Design review of the part built by this model. Coordinates are the model's own, in mm. Face numbers are marked on the shaded views. A direction names the side the tool comes from. Give positions to 0.01 mm unless a question says otherwise; leave off trailing zeros. Loops run counter-clockwise (first coordinate to the right, second up) from the corner with the lowest first, then second, coordinate; pieces in that order, holes last. Notation, with made-up numbers: M 18.5,-8 L 62.5,-8 A15 cw 62.5,17 Z; hole C 43,5 d2. An arc over 180 degrees is marked long. Use CSV: the item, a comma, the result in double quotes.
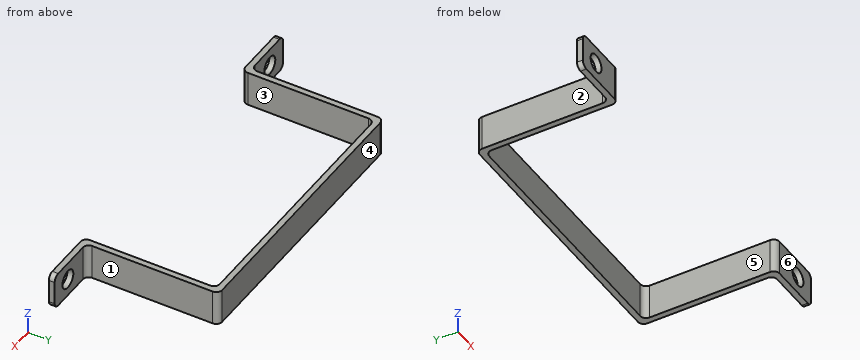
from build123d import *

# Parameters (mm, degrees)
EXTRUDE_1_DEPTH     = 12
FILLET_1_R          = 2
SKETCH_2_R          = 3.1
CUT_EXTRUDE_1_DEPTH = 12


with BuildPart() as part:
    # ｽｹｯﾁ1 → ﾎﾞｽ - 押し出し1 (new body)
    with BuildSketch(Plane.XY):
        Polygon((47, 0), (-47, 0), (-47, -45), (-65, -45), (-65, -47), (-45, -47), (-45, -2), (45, -2), (45, -47), (65, -47), (65, -45), (47, -45), align=None)
    extrude(amount=EXTRUDE_1_DEPTH)

    # ﾌｨﾚｯﾄ1
    fillet_1_edges = [part.edges().sort_by_distance(p)[0] for p in [
        (65, -46, 0),
        (-65, -46, 0),
        (-65, -46, 12),
        (45, -47, 6),
        (45, -2, 6),
        (-45, -2, 6),
        (-45, -47, 6),
        (-47, -45, 6),
        (-47, 0, 6),
        (47, 0, 6),
        (47, -45, 6),
        (65, -46, 12),
    ]]
    fillet(fillet_1_edges, radius=FILLET_1_R)

    # ｽｹｯﾁ2 → ｶｯﾄ - 押し出し1 (cut)
    with BuildSketch(Plane(origin=(0, -45, 0), x_dir=(1, 0, 0), z_dir=(0, 1, 0))):
        with Locations(Location((-57.5, -6, 0), (0, 0, 180))):
            Circle(SKETCH_2_R)
        with Locations(Location((57.5, -6, 0), (0, 0, 180))):
            Circle(SKETCH_2_R)
    extrude(amount=-CUT_EXTRUDE_1_DEPTH, mode=Mode.SUBTRACT)


solid = part.part
(1) The part is to be moulded in two halves that separate along X. For the marked faces 1, 2, 3 and 4, say which applies: released by +X, released by -X, zero draft, split by the parting line, or undercut.
A:
face 1,"released by +X"
face 2,"released by -X"
face 3,"undercut"
face 4,"zero draft"
(2) Machinability: for the marked faces 5 and 6, which of the approach directions +Z, -Z, +X, -X, +Y, -Y give a long, thin tool a straight path to every point of the face, cutting with its end or side? Answer none if there is none.
A:
face 5,"+Z, -Z, -Y"
face 6,"+Z, -Z, +X, -X, -Y"
(3) We need section B-B on x = -57.5. State the section outline as (y, z) points, then the cut area to 3 significant figures.
A:
outline,"M -47,0 L -45,0 L -45,2.9 L -47,2.9 Z; M -47,9.1 L -45,9.1 L -45,12 L -47,12 Z"
area,"11.6 mm²"
(4) We need section A-A on y = -37.5. State the section outline as (x, z) points, then the cut area to 3 significant figures.
A:
outline,"M -47,0 L -45,0 L -45,12 L -47,12 Z; M 45,0 L 47,0 L 47,12 L 45,12 Z"
area,"48.0 mm²"
(5) Clearance check with flat-ended pins moving along their axes: P1, Ø6, axis at x = 49.5, z = 4.5, coming from the +Y side; P2, Ø3.5, axis at y = -31, z = 4.5, coming from the -X side; P3, Ø3.5, axis at x = 60, z = 7.5, coming from the +Y side. State where each tip first meets the part, or that it passes through.
A:
P1,"y = -0.68"
P2,"x = -47"
P3,"y = -45"
(6) Wall thickness on line 1 along X through (y, z) = (-14, 3.75); line 2 along Z through (x, y) = (-57.5, -45.85); line 3 along Y through (x, z) = (-25.5, 2.75): over which ranges is each line inside the solid? List them lowest first. Write a range as [from, to].
A:
line 1,"[-47, -45], [45, 47]"
line 2,"[0, 2.9], [9.1, 12]"
line 3,"[-2, 0]"
